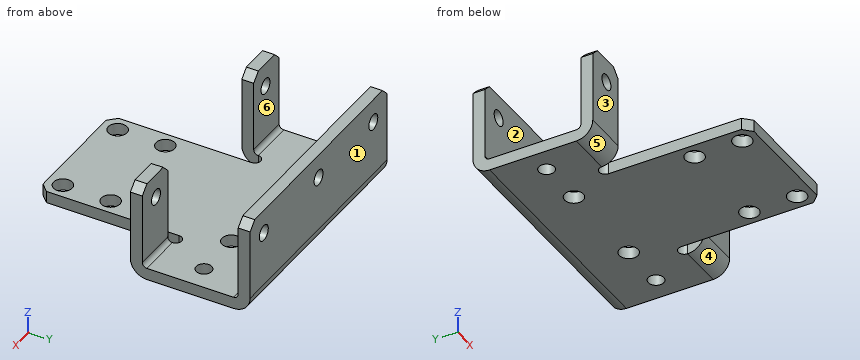
```python
from build123d import *

# Parameters (mm, degrees)
BOSS_EXTRUDE1_DEPTH        = 3.175
SKETCH2_W                  = 63.5
SKETCH2_H                  = 3.175
BOSS_EXTRUDE2_DEPTH        = 22.225
SKETCH3_W                  = 11.811
SKETCH3_H                  = 3.175
BOSS_EXTRUDE3_DEPTH        = 22.225
SKETCH4_W                  = 11.811
SKETCH4_H                  = 3.175
BOSS_EXTRUDE4_DEPTH        = 22.225
HOLE1_D                    = 4.9784
HOLE1_DEPTH                = 3.175
M3_5_CLEARANCE_HOLE1_D     = 4.1402
M3_5_CLEARANCE_HOLE1_DEPTH = 3.175
M3_5_CLEARANCE_HOLE2_D     = 4.1402
M3_5_CLEARANCE_HOLE2_DEPTH = 3.175
M3_5_CLEARANCE_HOLE3_D     = 4.1402
M3_5_CLEARANCE_HOLE3_DEPTH = 31.877
CHAMFER1_SIZE              = 2.159
FILLET1_R                  = 1.2192
FILLET2_R                  = 4.3942


with BuildPart() as part:
    # Sketch1 → Boss-Extrude1 (new body)
    with BuildSketch(Plane(origin=(0, 0, 0), x_dir=(-1, 0, 0), z_dir=(0, 0, -1))):
        with BuildLine():
            Line((-16.764, -49.0347), (16.764, -49.0347))
            Line((16.764, -49.0347), (16.764, -11.5443))
            ThreePointArc((16.764, -11.5443), (18.3515, -9.9568), (19.939, -11.5443))
            Line((19.939, -11.5443), (19.939, -15.9385))
            Line((19.939, -15.9385), (31.75, -15.9385))
            Line((31.75, -15.9385), (31.75, 15.9385))
            Line((31.75, 15.9385), (-31.75, 15.9385))
            Line((-31.75, 15.9385), (-31.75, -15.9385))
            Line((-31.75, -15.9385), (-19.939, -15.9385))
            Line((-19.939, -15.9385), (-19.939, -11.5443))
            ThreePointArc((-19.939, -11.5443), (-18.3515, -9.9568), (-16.764, -11.5443))
            Line((-16.764, -11.5443), (-16.764, -49.0347))
        make_face()
    extrude(amount=-BOSS_EXTRUDE1_DEPTH)

    # Sketch2 → Boss-Extrude2 (add)
    with BuildSketch(Plane.XY.offset(3.175)):
        with Locations((0, 14.351)):
            Rectangle(SKETCH2_W, SKETCH2_H)
    extrude(amount=BOSS_EXTRUDE2_DEPTH)

    # Sketch3 → Boss-Extrude3 (add)
    with BuildSketch(Plane.XY.offset(3.175)):
        with Locations((25.8445, -14.351)):
            Rectangle(SKETCH3_W, SKETCH3_H)
    extrude(amount=BOSS_EXTRUDE3_DEPTH)

    # Sketch4 → Boss-Extrude4 (add)
    with BuildSketch(Plane.XY.offset(3.175)):
        with Locations((-25.8445, -14.351)):
            Rectangle(SKETCH4_W, SKETCH4_H)
    extrude(amount=BOSS_EXTRUDE4_DEPTH)

    # Hole1
    with Locations(Plane.XY.offset(3.175)):
        with Locations((12.7, -44.831), (-12.7, -44.831), (-12.7, -32.131), (12.7, -32.131), (-12.7, 0), (12.7, 0)):
            Hole(HOLE1_D / 2, depth=HOLE1_DEPTH)

    # M3.5 Clearance Hole1
    with Locations(Plane.XY.offset(3.175)):
        with Locations((-25.4, 0), (25.4, 0)):
            Hole(M3_5_CLEARANCE_HOLE1_D / 2, depth=M3_5_CLEARANCE_HOLE1_DEPTH)

    # M3.5 Clearance Hole2
    with Locations(Plane(origin=(0, 15.9385, 0), x_dir=(1, 0, 0), z_dir=(0, 1, 0))):
        with Locations((25.4, -19.05), (0, -19.05), (-25.4, -19.05)):
            Hole(M3_5_CLEARANCE_HOLE2_D / 2, depth=M3_5_CLEARANCE_HOLE2_DEPTH)

    # M3.5 Clearance Hole3
    with Locations(Plane(origin=(0, -15.9385, 0), x_dir=(-1, 0, 0), z_dir=(0, -1, 0))):
        with Locations((-25.4, -19.05), (25.4, -19.05)):
            Hole(M3_5_CLEARANCE_HOLE3_D / 2, depth=M3_5_CLEARANCE_HOLE3_DEPTH)

    # Chamfer1
    chamfer1_edges = [part.edges().sort_by_distance(p)[0] for p in [
        (-19.939, -14.351, 25.4),
        (31.75, 14.351, 25.4),
        (31.75, -14.351, 25.4),
        (16.764, -49.0347, 1.5875),
        (-31.75, 14.351, 25.4),
        (-31.75, -14.351, 25.4),
        (19.939, -14.351, 25.4),
        (-16.764, -49.0347, 1.5875),
    ]]
    chamfer(chamfer1_edges, length=CHAMFER1_SIZE)

    # Fillet1
    fillet1_edges = [part.edges().sort_by_distance(p)[0] for p in [
        (25.8445, -12.7635, 3.175),
        (-25.8445, -12.7635, 3.175),
        (0, 12.7635, 3.175),
    ]]
    fillet(fillet1_edges, radius=FILLET1_R)

    # Fillet2
    fillet2_edges = [part.edges().sort_by_distance(p)[0] for p in [
        (25.8445, -15.9385, 0),
        (-25.8445, -15.9385, 0),
        (0, 15.9385, 0),
    ]]
    fillet(fillet2_edges, radius=FILLET2_R)


solid = part.part
```
The listing builds one solid part. Answer for the finished solid, in the listing's coordinates (mm). Face numbers are marked on the shaded views. A direction names the side the tool comes from. Coordinates: 2 decimals unless noted, no trailing zeros. Write each loop counter-clockwise with the first axis right and the second up, starting at its lowest first coordinate (ties: lowest second). Pieces come first, ordered by that corner, then holes. Notation, with made-up numbers: (21.25, 76) - (32.25, 76) arc R16 cw to (32.25, 97) - close; hole circle Ø1 at (38, -16.75). An arc over 180 degrees is marked (long way). Return JSON: item names as keys, results as strings. Group by question number.
1. Which of the six approach directions +Z, -Z, +X, -X, +Y, -Y give full straight-line access (tool end or side, diameter ignored) to the marked faces 4, 5 and 6?
2. A cutting plane is placed at C-C, the plane x = 5.5. Determine the outline of the cut face in (y, z) (1 decimal), plus the area to 3 significant figures.
3. A cutting plane is placed at A-A, the plane x = 12.7. Determine the outline of the cut face in (y, z) (1 decimal).
4. A cutting plane is placed at B-B, the plane z = 13.75. Determine the outline of the cut face in (x, y), plus the area to 3 significant figures.
5. Determine the mould class of the marked faces 1, 2 and 3 for opening direction Y: released by +Y, released by -Y, zero draft, split by the parting line, or undercut.
6. Given pin 1 (6 mm diameter, centred on x = -29, z = 19.5, fed in from -Y); pin 2 (3.5 mm diameter, centred on x = -25.4, z = 19.05, fed in from +Y); pin 3 (5.5 mm diameter, centred on x = -12.7, y = -44.831, fed in from +Z) (3 decimals), each flat-ended and moving along its own axis, determine where each tip first touches the part or whether it passes through.
7. Straight lines are drawn through the part: L1, parallel to X at y = 13.7, z = 19.05; L2, parallel to X at y = -15.15, z = 19.05; L3, parallel to Y at x = 12.7, z = 1.6. For each, find the intervals that lie inside material, in ascending order.
8. A cutting plane is placed at D-D, the plane y = -23. Determine the outline of the cut face in (x, z) (3 decimals), plus the area to 3 significant figures.
Ans:
{
 "1": {"face 4": "-Z, +X, -Y", "face 5": "-Z, -X, -Y", "face 6": "+Z, +X, -X"},
 "2": {"outline": "(-49, 0) - (11.5, 0) arc R4.4 ccw to (15.9, 4.4) - (15.9, 25.4) - (12.8, 25.4) - (12.8, 4.4) arc R1.2 cw to (11.5, 3.2) - (-49, 3.2) - close", "area": "273 mm²"},
 "3": {"outline": "(-49, 0) - (-47.3, 0) - (-47.3, 3.2) - (-49, 3.2) - close; (-42.3, 0) - (-34.6, 0) - (-34.6, 3.2) - (-42.3, 3.2) - close; (-29.6, 0) - (-2.5, 0) - (-2.5, 3.2) - (-29.6, 3.2) - close; (2.5, 0) - (11.5, 0) arc R4.4 ccw to (15.9, 4.4) - (15.9, 25.4) - (12.8, 25.4) - (12.8, 4.4) arc R1.2 cw to (11.5, 3.2) - (2.5, 3.2) - close"},
 "4": {"outline": "(-31.75, -15.94) - (-19.94, -15.94) - (-19.94, -12.76) - (-31.75, -12.76) - close; (-31.75, 12.76) - (31.75, 12.76) - (31.75, 15.94) - (-31.75, 15.94) - close; (19.94, -15.94) - (31.75, -15.94) - (31.75, -12.76) - (19.94, -12.76) - close", "area": "277 mm²"},
 "5": {"face 1": "released by +Y", "face 2": "undercut", "face 3": "released by -Y"},
 "6": {"pin 1": "y = -15.94", "pin 2": "through", "pin 3": "z = 3.175"},
 "7": {"L1": "-31.75 to -27.47, -23.33 to -2.07, 2.07 to 23.33, 27.47 to 31.75", "L2": "-31.75 to -27.47, -23.33 to -19.94, 19.94 to 23.33, 27.47 to 31.75", "L3": "-49.03 to -47.32, -42.34 to -34.62, -29.64 to -2.49, 2.49 to 14.94"},
 "8": {"outline": "(-16.764, 0) - (16.764, 0) - (16.764, 3.175) - (-16.764, 3.175) - close", "area": "106 mm²"}
}
